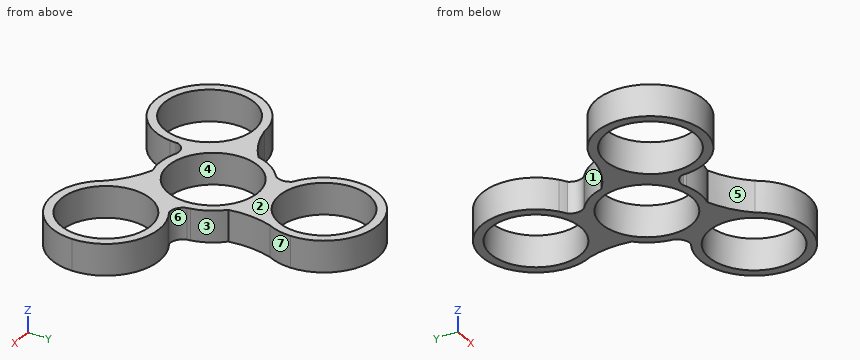
from build123d import *

# Parameters (mm, degrees)
F0_R     = 10
F1_DEPTH = 7
F2_DEPTH = 7


with BuildPart() as f1:
    # F0 (on Top) → F1 (new body)
    with BuildSketch(Plane.XY):
        with BuildLine():
            ThreePointArc((-7.905729, -12.970181), (-8.489375, -9.697228), (-9.948647, -6.710024))
            ThreePointArc((-9.948647, -6.710024), (-14.537703, -2.683439), (-20.514029, -1.435908))
            ThreePointArc((-20.514029, -1.435908), (-28.623409, -21.657457), (-7.968535, -14.725697))
            ThreePointArc((-7.968535, -14.725697), (-8.073222, -13.84307), (-7.905729, -12.970181))
        make_face()
        with Locations((-19.897294, -13.420049)):
            Circle(F0_R, mode=Mode.SUBTRACT)
        with BuildLine():
            ThreePointArc((11.882649, 1.674113), (11.805899, 2.006216), (11.768638, 2.34503))
            ThreePointArc((11.768638, 2.34503), (10.514847, 5.78256), (8.283423, 8.682448))
            ThreePointArc((8.283423, 8.682448), (4.070211, 11.288639), (-0.836728, 11.970793))
            ThreePointArc((-0.836728, 11.970793), (-4.302154, 11.202297), (-7.391149, 9.453619))
            ThreePointArc((-7.391149, 9.453619), (-7.640384, 9.2211), (-7.915175, 9.019424))
            ThreePointArc((-7.915175, 9.019424), (-10.265267, 6.214844), (-11.660932, 2.832431))
            ThreePointArc((-11.660932, 2.832431), (-11.811354, -2.119413), (-9.948647, -6.710024))
            ThreePointArc((-9.948647, -6.710024), (-7.550397, -9.326923), (-4.4915, -11.127732))
            ThreePointArc((-4.4915, -11.127732), (-4.165515, -11.227317), (-3.853463, -11.364454))
            ThreePointArc((-3.853463, -11.364454), (-0.24958, -11.997404), (3.377509, -11.514879))
            ThreePointArc((3.377509, -11.514879), (7.741143, -9.169226), (10.785375, -5.260768))
            ThreePointArc((10.785375, -5.260768), (11.692401, -2.699583), (12, 0))
            ThreePointArc((12, 0), (11.970626, 0.839111), (11.882649, 1.674113))
        make_face()
        Circle(F0_R, mode=Mode.SUBTRACT)
        with BuildLine():
            ThreePointArc((-9.948647, -6.710024), (-11.811354, -2.119413), (-11.660932, 2.832431))
            ThreePointArc((-11.660932, 2.832431), (-15.828168, 0.160413), (-20.514029, -1.435908))
            ThreePointArc((-20.514029, -1.435908), (-14.537703, -2.683439), (-9.948647, -6.710024))
        make_face()
    extrude(amount=F1_DEPTH)

    # F0 (on Top) → F2 (join)
    with BuildSketch(Plane.XY):
        with BuildLine():
            ThreePointArc((11.882649, 1.674113), (11.805899, 2.006216), (11.768638, 2.34503))
            ThreePointArc((11.768638, 2.34503), (10.514847, 5.78256), (8.283423, 8.682448))
            ThreePointArc((8.283423, 8.682448), (4.070211, 11.288639), (-0.836728, 11.970793))
            ThreePointArc((-0.836728, 11.970793), (-4.302154, 11.202297), (-7.391149, 9.453619))
            ThreePointArc((-7.391149, 9.453619), (-7.640384, 9.2211), (-7.915175, 9.019424))
            ThreePointArc((-7.915175, 9.019424), (-10.265267, 6.214844), (-11.660932, 2.832431))
            ThreePointArc((-11.660932, 2.832431), (-11.811354, -2.119413), (-9.948647, -6.710024))
            ThreePointArc((-9.948647, -6.710024), (-7.550397, -9.326923), (-4.4915, -11.127732))
            ThreePointArc((-4.4915, -11.127732), (-4.165515, -11.227317), (-3.853463, -11.364454))
            ThreePointArc((-3.853463, -11.364454), (-0.24958, -11.997404), (3.377509, -11.514879))
            ThreePointArc((3.377509, -11.514879), (7.741143, -9.169226), (10.785375, -5.260768))
            ThreePointArc((10.785375, -5.260768), (11.692401, -2.699583), (12, 0))
            ThreePointArc((12, 0), (11.970626, 0.839111), (11.882649, 1.674113))
        make_face()
        Circle(F0_R, mode=Mode.SUBTRACT)
        with BuildLine():
            ThreePointArc((11.882649, 1.674113), (11.8304, 2.01038), (11.768638, 2.34503))
            ThreePointArc((11.768638, 2.34503), (11.805899, 2.006216), (11.882649, 1.674113))
        make_face()
        with BuildLine():
            ThreePointArc((-0.836728, 11.970793), (4.070211, 11.288639), (8.283423, 8.682448))
            ThreePointArc((8.283423, 8.682448), (8.053006, 13.627389), (9.013482, 18.483624))
            ThreePointArc((9.013482, 18.483624), (4.944925, 13.931739), (-0.836728, 11.970793))
        make_face()
        with BuildLine():
            ThreePointArc((15.185371, -0.361472), (13.143603, 0.022889), (11.882649, 1.674113))
            ThreePointArc((11.882649, 1.674113), (11.970626, 0.839111), (12, 0))
            ThreePointArc((12, 0), (11.692401, -2.699583), (10.785375, -5.260768))
            ThreePointArc((10.785375, -5.260768), (12.642734, -2.5034), (15.185371, -0.361472))
        make_face()
        with BuildLine():
            ThreePointArc((-7.391149, 9.453619), (-4.302154, 11.202297), (-0.836728, 11.970793))
            ThreePointArc((-0.836728, 11.970793), (-4.153358, 12.200628), (-7.279641, 13.331653))
            ThreePointArc((-7.279641, 13.331653), (-6.591624, 11.37125), (-7.391149, 9.453619))
        make_face()
        with BuildLine():
            ThreePointArc((-7.279641, 13.331653), (-4.153358, 12.200628), (-0.836728, 11.970793))
            ThreePointArc((-0.836728, 11.970793), (4.944925, 13.931739), (9.013482, 18.483624))
            ThreePointArc((9.013482, 18.483624), (9.993661, 21.134743), (10.326544, 23.941586))
            ThreePointArc((10.326544, 23.941586), (-7.098341, 34.645353), (-8.768561, 14.263803))
            ThreePointArc((-8.768561, 14.263803), (-7.951839, 13.913151), (-7.279641, 13.331653))
        make_face()
        with Locations((-1.673456, 23.941586)):
            Circle(F0_R, mode=Mode.SUBTRACT)
        with BuildLine():
            ThreePointArc((16.737096, 0.461895), (16.025062, -0.07008), (15.185371, -0.361472))
            ThreePointArc((15.185371, -0.361472), (12.642734, -2.5034), (10.785375, -5.260768))
            ThreePointArc((10.785375, -5.260768), (9.592778, -11.248299), (11.500547, -17.047716))
            ThreePointArc((11.500547, -17.047716), (24.973511, -22.028979), (33.57075, -10.521537))
            ThreePointArc((33.57075, -10.521537), (28.128042, -0.471566), (16.737096, 0.461895))
        make_face()
        with Locations((21.57075, -10.521537)):
            Circle(F0_R, mode=Mode.SUBTRACT)
        with BuildLine():
            ThreePointArc((16.737096, 0.461895), (15.946147, 0.078644), (15.185371, -0.361472))
            ThreePointArc((15.185371, -0.361472), (16.025062, -0.07008), (16.737096, 0.461895))
        make_face()
        with BuildLine():
            ThreePointArc((-7.915175, 9.019424), (-7.640384, 9.2211), (-7.391149, 9.453619))
            ThreePointArc((-7.391149, 9.453619), (-7.65624, 9.240237), (-7.915175, 9.019424))
        make_face()
        with BuildLine():
            ThreePointArc((-8.768561, 14.263803), (-8.041181, 13.770446), (-7.279641, 13.331653))
            ThreePointArc((-7.279641, 13.331653), (-7.951839, 13.913151), (-8.768561, 14.263803))
        make_face()
        with BuildLine():
            ThreePointArc((11.500547, -17.047716), (9.592778, -11.248299), (10.785375, -5.260768))
            ThreePointArc((10.785375, -5.260768), (7.741143, -9.169226), (3.377509, -11.514879))
            ThreePointArc((3.377509, -11.514879), (7.775162, -13.787802), (11.500547, -17.047716))
        make_face()
        with BuildLine():
            ThreePointArc((-9.948647, -6.710024), (-11.811354, -2.119413), (-11.660932, 2.832431))
            ThreePointArc((-11.660932, 2.832431), (-15.828168, 0.160413), (-20.514029, -1.435908))
            ThreePointArc((-20.514029, -1.435908), (-14.537703, -2.683439), (-9.948647, -6.710024))
        make_face()
        with BuildLine():
            ThreePointArc((-4.4915, -11.127732), (-4.17416, -11.250617), (-3.853463, -11.364454))
            ThreePointArc((-3.853463, -11.364454), (-4.165515, -11.227317), (-4.4915, -11.127732))
        make_face()
        with BuildLine():
            ThreePointArc((-4.4915, -11.127732), (-7.550397, -9.326923), (-9.948647, -6.710024))
            ThreePointArc((-9.948647, -6.710024), (-8.489375, -9.697228), (-7.905729, -12.970181))
            ThreePointArc((-7.905729, -12.970181), (-6.551979, -11.394139), (-4.4915, -11.127732))
        make_face()
        with BuildLine():
            ThreePointArc((-7.905729, -12.970181), (-8.489375, -9.697228), (-9.948647, -6.710024))
            ThreePointArc((-9.948647, -6.710024), (-14.537703, -2.683439), (-20.514029, -1.435908))
            ThreePointArc((-20.514029, -1.435908), (-28.623409, -21.657457), (-7.968535, -14.725697))
            ThreePointArc((-7.968535, -14.725697), (-8.073222, -13.84307), (-7.905729, -12.970181))
        make_face()
        with Locations((-19.897294, -13.420049)):
            Circle(F0_R, mode=Mode.SUBTRACT)
        with BuildLine():
            ThreePointArc((-7.897294, -13.420049), (-7.899403, -13.195075), (-7.905729, -12.970181))
            ThreePointArc((-7.905729, -12.970181), (-8.073222, -13.84307), (-7.968535, -14.725697))
            ThreePointArc((-7.968535, -14.725697), (-7.915117, -14.073844), (-7.897294, -13.420049))
        make_face()
    extrude(amount=F2_DEPTH)


solid = f1.part
Here's how the part is built. I have some questions about the finished solid (model axes, mm). Face numbers are marked on the shaded views. A direction names the side the tool comes from. Coordinates: 2 decimals unless noted, no trailing zeros. Order: outer loops, then holes, each group sorted by start corner. A loop starts at its lowest first (then second) coordinate and runs counter-clockwise, first axis right, second up. Notation, with made-up numbers: (32.5, 87.5) -> (51.5, 87.5) arc R24 cw to (51.5, 101.5) -> close; hole circle Ø9 at (74, 46.25). An arc over 180 degrees is marked (long way). Answer in a Markdown table with one row per item.
(1) I want a section at C-C on y = -16. List the corners of the cut face in (x, z) for me.
Answer key:
| item | result |
|---|---|
| outline | (-31.62, 0) -> (-29.56, 0) -> (-29.56, 7) -> (-31.62, 7) -> close; (-10.24, 0) -> (-8.18, 0) -> (-8.18, 7) -> (-10.24, 7) -> close; (10.49, 0) -> (13.2, 0) -> (13.2, 7) -> (10.49, 7) -> close; (29.94, 0) -> (32.25, 0) -> (32.25, 7) -> (29.94, 7) -> close |
(2) I want a section at D-D on y = 25. List the corners of the cut face in (x, z) for me, then the cut area to 3 significant figures.
Answer key:
| item | result |
|---|---|
| outline | (-13.63, 0) -> (-11.62, 0) -> (-11.62, 7) -> (-13.63, 7) -> close; (8.27, 0) -> (10.28, 0) -> (10.28, 7) -> (8.27, 7) -> close |
| area | 28.1 mm^2 |
(3) Thinking about a two-plate mould opening in X: for the marked faces 1, 2, 3 and 4, which applies, +X half, -X half, draft (parallel to the pull), parting line (faces both ways), or undercut?
Answer key:
| item | result |
|---|---|
| face 1 | -X half |
| face 2 | draft |
| face 3 | +X half |
| face 4 | undercut |
(4) I want a section at B-B on z = 3. List the corners of the cut face in (x, y) for me.
Answer key:
| item | result |
|---|---|
| outline | (-20.51, -1.44) arc R12 ccw (long way) to (-7.97, -14.73) arc R12 ccw to (-7.9, -13.42) arc R12 ccw to (-7.91, -12.97) arc R2.9 cw to (-4.49, -11.13) arc R12 ccw to (-3.85, -11.36) arc R12 ccw to (3.38, -11.51) arc R20.52 cw to (11.5, -17.05) arc R12 ccw (long way) to (16.74, 0.46) arc R12 ccw to (15.19, -0.36) arc R2.9 cw to (11.88, 1.67) arc R12 ccw to (11.77, 2.35) arc R12 ccw to (8.28, 8.68) arc R20.52 cw to (9.01, 18.48) arc R12 ccw to (10.33, 23.94) arc R12 ccw (long way) to (-8.77, 14.26) arc R12 ccw to (-7.28, 13.33) arc R2.9 cw to (-7.39, 9.45) arc R12 ccw to (-7.92, 9.02) arc R12 ccw to (-11.66, 2.83) arc R20.52 cw to start; hole circle Ø20 at (-19.9, -13.42); hole circle Ø20 at (-1.67, 23.94); hole circle Ø20 at (0, 0); hole circle Ø20 at (21.57, -10.52) |
(5) On a 3-axis mill with a long thin cutter (end or side, diameter ignored), from which of +Z, -Z, +X, -X, +Y, -Y can I reach the whole of each face in a straight line? I mean the marked faces 5, 6 and 7. Say none if no direction works.
Answer key:
| item | result |
|---|---|
| face 5 | +Z, -Z, -Y |
| face 6 | +Z, -Z, +Y |
| face 7 | +Z, -Z, +X |
(6) Will these pins go through, and if not, where does the flat tip stop? pin 1 Ø18 at (x, y) = (-19.9, -13.42) entering from +Z; pin 2 Ø2 at (x, z) = (-7.5, 1.5) entering from +Y; pin 3 Ø2 at (x, z) = (-20, 1) entering from +Y; pin 4 Ø2 at (y, z) = (1, 6.5) entering from -X.
Answer key:
| item | result |
|---|---|
| pin 1 | through |
| pin 2 | y = 34.93 |
| pin 3 | y = -1.06 |
| pin 4 | x = -16.17 |
(7) Please list where these lines run through material, in increasing order: probe 1 along Y at (x, z) = (5.5, 3.5); probe 2 along X at (y, z) = (-8.5, 6); probe 3 along X at (y, z) = (-11, 3).
Answer key:
| item | result |
|---|---|
| probe 1 | -12.44 to -8.35, 8.35 to 16.97, 30.91 to 33.56 |
| probe 2 | -30.84 to -28.6, -11.19 to -5.27, 5.27 to 11.78, 31.36 to 33.4 |
| probe 3 | -31.65 to -29.6, -10.19 to 11.58, 31.56 to 33.56 |
(8) I want a section at A-A on x = 23. List the corners of the cut face in (y, z) for me, then the cut area to 3 significant figures.
Answer key:
| item | result |
|---|---|
| outline | (-22.44, 0) -> (-20.42, 0) -> (-20.42, 7) -> (-22.44, 7) -> close; (-0.62, 0) -> (1.39, 0) -> (1.39, 7) -> (-0.62, 7) -> close |
| area | 28.2 mm^2 |
